Check sheet for the modelled part. Datum: model origin and axes. Units: mm. A direction names the side the tool comes from. Round coordinates to 2 decimals unless told otherwise and drop trailing zeros. Order: outer loops, then holes, each group sorted by start corner. A loop starts at its lowest first (then second) coordinate and runs counter-clockwise, first axis right, second up. Notation, with made-up numbers: (55.25, -19.75) -> (110.25, -19.75) arc R10 ccw to (110.25, -11.75) -> close; hole circle Ø5 at (-9.5, 19). An arc over 180 degrees is marked (long way). Answer in a Markdown table with one row per item. Add a question column.
1. Access from +Z, -Z, +X, -X, +Y, -Y to the whole of each face (thin tool, end or side, straight path). Record for faces 1 (the cylindrical face through (7.1, 0, 2)), 2 (the cylindrical face through (-11.987, -12.189, 2.113)), 3 (the flat face through (0.2, -13.7, 0.5)).
2. Material ranges on L1, parallel to Y at x = 0, z = 2; L2, parallel to Z at x = -11, y = 3; L3, parallel to Z at x = 2, y = 10, recorded low to high. Write a range as from..to.
3. Sectioned sample at B-B, the plane x = 8.2. Record the boundary of the cut face in (y, z).
4. Sectioned sample at C-C, the plane y = 7.1. Record the boundary of the cut face in (x, z).
5. Draft check along X on faces 4 (the cylindrical face through (15.647, -13.559, 1.521)), 5 (the flat face through (5, -10, 11)), 6 (the cylindrical face through (-12.819, 18.503, 2.113)). Enter one of: +X half, -X half, draft (parallel to the pull), parting line (faces both ways), or undercut.
6. Sectioned sample at D-D, the plane x = -5.5. Record the boundary of the cut face in (y, z), then the cut area to 3 significant figures.
7. Sectioned sample at A-A, the plane y = 0. Record the boundary of the cut face in (x, z), then the cut area to 3 significant figures.
8. Depth check by flat-ended pin: P1, Ø1.5, axis at y = 4.5, z = 7, coming from the +X side; P2, Ø4, axis at x = -14.5, y = -12, coming from the +Z side; P3, Ø8, axis at x = 6.5, y = -10.5, coming from the -Z side; P4, Ø1.5, axis at x = -8, y = 7, coming from the -Z side. Enter the tip coordinate at first touch or a pass-through.
```python
from build123d import *

# Parameters (mm, degrees)
SZKIC1_R                    = 3
SZKIC1_R_2                  = 1.1
SZKIC1_R_3                  = 1
DODANIE_WYCI_GNI_CIE1_DEPTH = 3
SZKIC2_R                    = 12
SZKIC2_R_2                  = 11
DODANIE_WYCI_GNI_CIE2_DEPTH = 8
SZKIC3_R                    = 1.1
SZKIC3_R_2                  = 3
WYTNIJ_WYCI_GNI_CIE1_DEPTH  = 1
SZKIC4_R                    = 1.8
WYTNIJ_WYCI_GNI_CIE2_DEPTH  = 1.8
ZAOKR_GLENIE1_R             = 4


with BuildPart() as part:
    # Szkic1 → Dodanie-wyciągnięcie1 (new body)
    with BuildSketch(Plane.XY):
        Polygon((-16.85, 0), (-16.85, -14.7), (0, -14.7), (16.85, -14.7), (16.85, 23.3), (-16.85, 23.3), align=None)
        Circle(SZKIC1_R, mode=Mode.SUBTRACT)
        with Locations((-8.2, 0)):
            Circle(SZKIC1_R_2, mode=Mode.SUBTRACT)
        with Locations((8.2, 0)):
            Circle(SZKIC1_R_2, mode=Mode.SUBTRACT)
        with Locations((0, 7.1)):
            Circle(SZKIC1_R_2, mode=Mode.SUBTRACT)
        with Locations((0, -7.1)):
            Circle(SZKIC1_R_2, mode=Mode.SUBTRACT)
        with Locations((-13.65, 20.1)):
            Circle(SZKIC1_R_3, mode=Mode.SUBTRACT)
        with Locations((13.65, 20.1)):
            Circle(SZKIC1_R_3, mode=Mode.SUBTRACT)
        with Locations((13.65, -11.5)):
            Circle(SZKIC1_R_3, mode=Mode.SUBTRACT)
        with Locations((-13.65, -11.5)):
            Circle(SZKIC1_R_3, mode=Mode.SUBTRACT)
    extrude(amount=DODANIE_WYCI_GNI_CIE1_DEPTH)

    # Szkic2 → Dodanie-wyciągnięcie2 (add)
    with BuildSketch(Plane.XY.offset(3)):
        Circle(SZKIC2_R)
        Circle(SZKIC2_R_2, mode=Mode.SUBTRACT)
    extrude(amount=DODANIE_WYCI_GNI_CIE2_DEPTH)

    # Szkic3 → Wytnij-wyciągnięcie1 (cut)
    with BuildSketch(Plane(origin=(0, 0, 0), x_dir=(-1, 0, 0), z_dir=(0, 0, -1))):
        with BuildLine():
            Line((11.326209992, 22.3), (-11.326209992, 22.3))
            ThreePointArc((-11.326209992, 22.3), (-10.67711184, 21.284033778), (-10.45, 20.1))
            ThreePointArc((-10.45, 20.1), (-12.385088936, 17.160612309), (-15.85, 17.776209992))
            Line((-15.85, 17.776209992), (-15.85, -9.176209992))
            ThreePointArc((-15.85, -9.176209992), (-12.385088936, -8.560612309), (-10.45, -11.5))
            ThreePointArc((-10.45, -11.5), (-10.67711184, -12.684033778), (-11.326209992, -13.7))
            Line((-11.326209992, -13.7), (11.326209992, -13.7))
            ThreePointArc((11.326209992, -13.7), (11.3872583, -9.2372583), (15.85, -9.176209992))
            Line((15.85, -9.176209992), (15.85, 17.776209992))
            ThreePointArc((15.85, 17.776209992), (11.3872583, 17.8372583), (11.326209992, 22.3))
        make_face()
        with Locations((-8.2, 0)):
            Circle(SZKIC3_R, mode=Mode.SUBTRACT)
        with Locations((0, -7.1)):
            Circle(SZKIC3_R, mode=Mode.SUBTRACT)
        Circle(SZKIC3_R_2, mode=Mode.SUBTRACT)
        with Locations((8.2, 0)):
            Circle(SZKIC3_R, mode=Mode.SUBTRACT)
        with Locations((0, 7.1)):
            Circle(SZKIC3_R, mode=Mode.SUBTRACT)
    extrude(amount=-WYTNIJ_WYCI_GNI_CIE1_DEPTH, mode=Mode.SUBTRACT)

    # Szkic4 → Wytnij-wyciągnięcie2 (cut)
    with BuildSketch(Plane.XY.offset(3)):
        with Locations((-13.65, 20.1)):
            Circle(SZKIC4_R)
        with Locations((13.65, 20.1)):
            Circle(SZKIC4_R)
        with Locations((13.65, -11.5)):
            Circle(SZKIC4_R)
        with Locations((-13.65, -11.5)):
            Circle(SZKIC4_R)
    extrude(amount=-WYTNIJ_WYCI_GNI_CIE2_DEPTH, mode=Mode.SUBTRACT)

    # Zaokrąglenie1
    zaokr_glenie1_edges = [part.edges().sort_by_distance(p)[0] for p in [
        (-16.85, 23.3, 1.5),
        (16.85, 23.3, 1.5),
        (16.85, -14.7, 1.5),
        (-16.85, -14.7, 1.5),
    ]]
    fillet(zaokr_glenie1_edges, radius=ZAOKR_GLENIE1_R)


solid = part.part
```
Answer key:
| question | item | result |
|---|---|---|
| 1 | face 1 | +Z, -Z |
| 1 | face 2 | +Z |
| 1 | face 3 | -Z |
| 2 | L1 | y = -14.7..-8.2, -6..-3, 3..6, 8.2..23.3 |
| 2 | L2 | z = 1..11 |
| 2 | L3 | z = 1..3 |
| 3 | outline | (-14.7, 0) -> (-13.7, 0) -> (-13.7, 1) -> (-1.1, 1) -> (-1.1, 3) -> (-7.33, 3) -> (-7.33, 11) -> (-8.76, 11) -> (-8.76, 3) -> (-14.7, 3) -> close; (1.1, 1) -> (22.3, 1) -> (22.3, 0) -> (23.3, 0) -> (23.3, 3) -> (8.76, 3) -> (8.76, 11) -> (7.33, 11) -> (7.33, 3) -> (1.1, 3) -> close |
| 4 | outline | (-16.85, 0) -> (-15.85, 0) -> (-15.85, 1) -> (-1.1, 1) -> (-1.1, 3) -> (-8.4, 3) -> (-8.4, 11) -> (-9.67, 11) -> (-9.67, 3) -> (-16.85, 3) -> close; (1.1, 1) -> (15.85, 1) -> (15.85, 0) -> (16.85, 0) -> (16.85, 3) -> (9.67, 3) -> (9.67, 11) -> (8.4, 11) -> (8.4, 3) -> (1.1, 3) -> close |
| 5 | face 4 | +X half |
| 5 | face 5 | draft |
| 5 | face 6 | undercut |
| 6 | outline | (-14.7, 0) -> (-13.7, 0) -> (-13.7, 1) -> (22.3, 1) -> (22.3, 0) -> (23.3, 0) -> (23.3, 3) -> (10.67, 3) -> (10.67, 11) -> (9.53, 11) -> (9.53, 3) -> (-9.53, 3) -> (-9.53, 11) -> (-10.67, 11) -> (-10.67, 3) -> (-14.7, 3) -> close |
| 6 | area | 96.2 mm² |
| 7 | outline | (-16.85, 0) -> (-15.85, 0) -> (-15.85, 1) -> (-9.3, 1) -> (-9.3, 3) -> (-11, 3) -> (-11, 11) -> (-12, 11) -> (-12, 3) -> (-16.85, 3) -> close; (-7.1, 1) -> (-3, 1) -> (-3, 3) -> (-7.1, 3) -> close; (3, 1) -> (7.1, 1) -> (7.1, 3) -> (3, 3) -> close; (9.3, 1) -> (15.85, 1) -> (15.85, 0) -> (16.85, 0) -> (16.85, 3) -> (12, 3) -> (12, 11) -> (11, 11) -> (11, 3) -> (9.3, 3) -> close |
| 7 | area | 64.6 mm² |
| 8 | P1 | stops at x = 11.4 |
| 8 | P2 | stops at z = 3 |
| 8 | P3 | stops at z = 0 |
| 8 | P4 | stops at z = 1 |
